Geometry check sheet. Reference: the model listing, model coordinates, mm. Face numbers are marked on the shaded views. A direction names the side the tool comes from. Give positions to 0.01 mm unless a question says otherwise; leave off trailing zeros. Order: outer loops, then holes, each group sorted by start corner. A loop starts at its lowest first (then second) coordinate and runs counter-clockwise, first axis right, second up. Notation, with made-up numbers: M 16,71.25 L 27,71.25 A15 cw 27,76.25 Z; hole C 65,-38 d9. An arc over 180 degrees is marked long. Answer as CSV lines item,"result". Start each with the question number.
Q1. Section check C-C, the plane x = 0.5. Record the boundary of the cut face in (y, z).
Q2. Set-up check for the marked faces 4, 5 and 6: record each of +Z, -Z, +X, -X, +Y, -Y from which the full face is reachable in a straight line by a thin tool's end or side.
Q3. Mould release check, pull along X, two halves, no side actions. Record for the marked faces 1, 2 and 3: +X half, -X half, draft (parallel to the pull), parting line (faces both ways), or undercut.
Q4. Go/stop test with flat-tipped pins: pin 1 (1.5 mm diameter, centred on x = 0, z = -0.5, fed in from +Y); pin 2 (1 mm diameter, centred on x = -2, y = 8.5, fed in from +Z); pin 3 (0.6 mm diameter, centred on x = -2, y = 9.5, fed in from -Z); pin 4 (1.6 mm diameter, centred on x = 0, z = 0, fed in from +Y). Record where each tip stops, or that it passes through.
Q5. Section check B-B, the plane x = -2. Record the boundary of the cut face in (y, z).
Q6. Section check D-D, the plane y = 14. Record the boundary of the cut face in (x, z), then the cut area to 3 significant figures.
Q7. Section check A-A, the plane z = 0. Record the boundary of the cut face in (x, y), then the cut area to 3 significant figures.
Q8. Thickness scan on line 1 (Z direction, x = 0, y = 11.5); line 2 (Z direction, x = 0, y = 3.2); line 3 (X direction, y = 13.25, z = -0.5). Record the ranges inside material, lowest first.
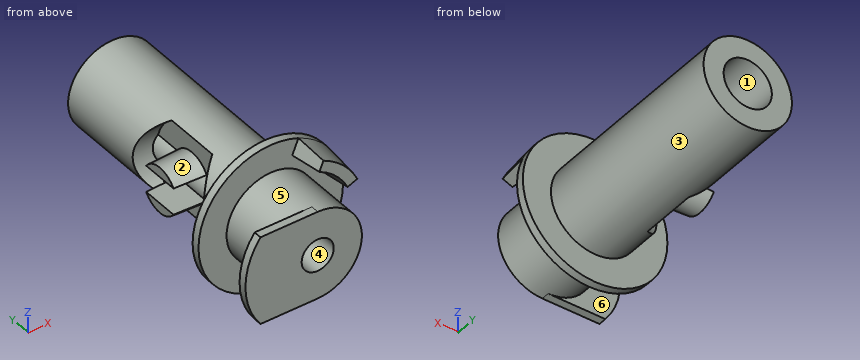
```python
from build123d import *

# Parameters (mm, degrees)
SKETCH_1_R                = 4.5
EXTRUDE_1_DEPTH           = 17.5
SKETCH_2_W                = 1.75
SKETCH_2_H                = 13
SKETCH_3_W                = 1.75
SKETCH_3_H                = 3.5
CUT_EXTRUDE_1_DEPTH       = 0.5
EXTRUDE_2_DEPTH           = 2
EXTRUDE_2_DRAFT           = 5
SKETCH_7_R                = 3
CUT_EXTRUDE_2_DEPTH       = 1.5
SKETCH_8_R                = 1.5
EXTRUDE_3_DEPTH           = 2
EXTRUDE_3_TAPER           = 2
HOLE_WIZARD_1_D           = 2
HOLE_WIZARD_1_CBORE_D     = 3
HOLE_WIZARD_1_CBORE_DEPTH = 13
CUT_EXTRUDE_4_REACH       = 9.75
SKETCH_16_W               = 1.658312396
SKETCH_16_H               = 2.982539584


with BuildPart() as part:
    # 草图1 → 凸台-拉伸1 (new body)
    with BuildSketch(Plane(origin=(0, 0, 0), x_dir=(1, 0, 0), z_dir=(0, 1, 0))):
        Circle(SKETCH_1_R)
    extrude(amount=EXTRUDE_1_DEPTH)

    # 草图2 → 切除-旋转1 (revolve, cut)
    with BuildSketch(Plane.XY):
        with Locations((3.625, 11)):
            Rectangle(SKETCH_2_W, SKETCH_2_H)
    revolve(axis=Axis((0, 0, 0), (0, -1, 0)), mode=Mode.SUBTRACT)

    # 草图3 → 切除-旋转2 (revolve, cut)
    with BuildSketch(Plane.XY):
        with Locations((3.625, 2.25)):
            Rectangle(SKETCH_3_W, SKETCH_3_H)
    revolve(axis=Axis((0, 0, 0), (0, 1, 0)), mode=Mode.SUBTRACT)

    # 草图4 → 切除-拉伸1 (cut)
    with BuildSketch(Plane.XZ):
        with BuildLine():
            Line((0, 2.75), (-3.561951712, 2.75))
            ThreePointArc((-3.561951712, 2.75), (4.5, 0), (-3.561951712, -2.75))
            Line((-3.561951712, -2.75), (0, -2.75))
            ThreePointArc((0, -2.75), (2.75, 0), (0, 2.75))
        make_face()
    extrude(amount=-CUT_EXTRUDE_1_DEPTH, mode=Mode.SUBTRACT)


with BuildPart() as extrude_2_tool:
    # 草图6 → 凸台-拉伸2 (with draft: the straight prism first)
    with BuildSketch(Plane.XZ.offset(-4)):
        with BuildLine():
            ThreePointArc((1.339392013, 3.233578364), (2.474873734, 2.474873734), (3.233578364, 1.339392013))
            Line((3.233578364, 1.339392013), (4.157457896, 1.722075446))
            ThreePointArc((4.157457896, 1.722075446), (3.181980515, 3.181980515), (1.722075446, 4.157457896))
            Line((1.722075446, 4.157457896), (1.339392013, 3.233578364))
        make_face()
    extrude(amount=EXTRUDE_2_DEPTH)
    # 凸台-拉伸2: the draft: its side faces are tilted about the plane it starts from
    extrude_2_sides = [extrude_2_tool.faces().sort_by_distance(p)[0] for p in [
        (3.181980515, 3, 3.181980515),
        (1.530733729, 3, 3.69551813),
        (2.474873734, 3, 2.474873734),
        (3.69551813, 3, 1.530733729),
    ]]
    draft(extrude_2_sides, Plane.XZ.offset(-4), EXTRUDE_2_DRAFT)


with BuildPart() as part_1:
    add(part.part)

    # 凸台-拉伸2: add extrude_2_tool
    add(extrude_2_tool.part)

    # 草图7 → 切除-拉伸2 (cut)
    with BuildSketch(Plane(origin=(-2.75, 0, 0), x_dir=(0, 0, -1), z_dir=(1, 0, 0))):
        with Locations((0, 9)):
            Circle(SKETCH_7_R)
    extrude(amount=CUT_EXTRUDE_2_DEPTH, mode=Mode.SUBTRACT)

    # 草图8 → 凸台-拉伸3 (add)
    with BuildSketch(Plane.ZY.offset(1.25)):
        with Locations((0, 9)):
            Circle(SKETCH_8_R)
    extrude(amount=EXTRUDE_3_DEPTH, taper=EXTRUDE_3_TAPER)

    # 孔1 (through all)
    with Locations(Plane(origin=(0, 17.5, 0), x_dir=(1, 0, 0), z_dir=(0, 1, 0))):
        with Locations((0, 0)):
            CounterBoreHole(HOLE_WIZARD_1_D / 2, HOLE_WIZARD_1_CBORE_D / 2, HOLE_WIZARD_1_CBORE_DEPTH)

    # 草图16 → 切除-拉伸4 (cut, up to next)
    with BuildSketch(Plane.ZY.offset(3.25), mode=Mode.PRIVATE) as cut_extrude_4_sk1:
        with Locations((0, 9)):
            Rectangle(SKETCH_16_W, SKETCH_16_H)
    cut_extrude_4_tool1 = extrude(cut_extrude_4_sk1.sketch, amount=-CUT_EXTRUDE_4_REACH, mode=Mode.PRIVATE) & part_1.part
    add(cut_extrude_4_tool1.solids().sort_by_distance((-3.25, 9, 0))[0], mode=Mode.SUBTRACT)


solid = part_1.part
```
Answer block:
1,outline,"M 0,-2.7 L 4,-2.7 L 4,-4.47 L 4.5,-4.47 L 4.5,-2.7 L 17.5,-2.7 L 17.5,-1.41 L 4.5,-1.41 L 4.5,-0.87 L 0,-0.87 Z; M 0,0.87 L 4.5,0.87 L 4.5,1.41 L 17.5,1.41 L 17.5,2.7 L 4.5,2.7 L 4.5,4.47 L 4,4.47 L 4,2.7 L 0,2.7 Z"
2,face 4,"+Y, -Y"
2,face 5,"none"
2,face 6,"-X"
3,face 1,"undercut"
3,face 2,"-X half"
3,face 3,"parting line"
4,pin 1,"stops at y = 4.5"
4,pin 2,"stops at z = 1.48"
4,pin 3,"stops at z = -1.46"
4,pin 4,"passes through"
5,outline,"M 0,-2.75 L 0.5,-2.75 L 0.5,-1.89 L 4,-1.89 L 4,-4.03 L 4.5,-4.03 L 4.5,-1.89 L 6.67,-1.89 A3 cw 6.67,1.89 L 4.5,1.89 L 4.5,4.03 L 4,4.03 L 4,1.89 L 0.5,1.89 L 0.5,2.75 L 0,2.75 Z; M 7.78,-0.83 A1.47 ccw 10.22,-0.83 Z; M 7.78,0.83 L 10.22,0.83 A1.47 ccw Z; M 11.33,-1.89 L 17.5,-1.89 L 17.5,1.89 L 11.33,1.89 A3 cw Z"
6,outline,"C 0,0 d5.5; hole C 0,0 d3"
6,area,"16.7 mm2"
7,outline,"M -4.5,0 L -1,0 L -1,4.5 L -1.5,4.5 L -1.5,6 L -2.75,6 L -2.75,4.5 L -4.5,4.5 L -4.5,4 L -2.75,4 L -2.75,0.5 L -4.5,0.5 Z; M -2.75,12 L -1.5,12 L -1.5,17.5 L -2.75,17.5 Z; M 1,0 L 2.75,0 L 2.75,4 L 4.5,4 L 4.5,4.5 L 2.75,4.5 L 2.75,17.5 L 1.5,17.5 L 1.5,4.5 L 1,4.5 Z"
7,area,"43.4 mm2"
8,line 1,"z = -2.75 to -1.5, 1.5 to 2.75"
8,line 2,"z = -2.75 to -1, 1 to 2.75"
8,line 3,"x = -2.7 to -1.41, 1.41 to 2.7"
